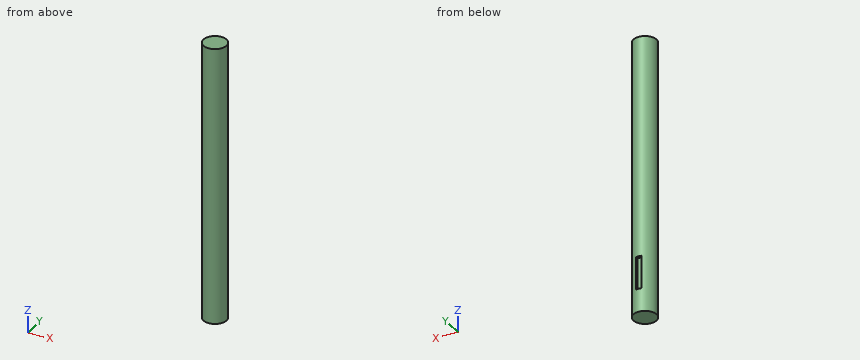
from build123d import *

# Parameters (mm, degrees)
SKETCH1_R           = 6.35
BOSS_EXTRUDE1_DEPTH = 152.4
CUT_EXTRUDE1_DEPTH  = 18.034


with BuildPart() as part:
    # Sketch1 → Boss-Extrude1 (new body)
    with BuildSketch(Plane.XY):
        with Locations(Location((0, 0, 0), (0, 0, 180))):
            Circle(SKETCH1_R)
    extrude(amount=BOSS_EXTRUDE1_DEPTH)

    # Sketch2 → Cut-Extrude1 (cut)
    with BuildSketch(Plane(origin=(0, 0, 12.7), x_dir=(-1, 0, 0), z_dir=(0, 0, -1))):
        Polygon((1.571433325, 4.7625), (-0.016066675, 4.7625), (-1.603566675, 4.7625), (-1.603566675, 7.9375), (1.571433325, 7.9375), align=None)
    extrude(amount=-CUT_EXTRUDE1_DEPTH, mode=Mode.SUBTRACT)


solid = part.part
Part model, mm, in its own coordinate system. Give positions to 0.01 mm unless a question says otherwise; leave off trailing zeros. Write each loop counter-clockwise with the first axis right and the second up, starting at its lowest first coordinate (ties: lowest second). Pieces come first, ordered by that corner, then holes.
1) Cut at A-A on z = 129. Write the cut outline in (x, y).
Resolved:
outline: circle Ø12.7 at (0, 0)
2) Probe L1, parallel to Y at x = 0.5, z = 121.5; L2, parallel to X at y = -4.5, z = 93.5; L3, parallel to Y at x = 2.5, z = 79. List the from-to ranges inside material, lowest first.
Resolved:
L1: y = -6.33 to 6.33
L2: x = -4.48 to 4.48
L3: y = -5.84 to 5.84
3) Cut at C-C on y = -3.25. Write the cut outline in (x, z), then the cut area to 3 significant figures.
Resolved:
outline: (-5.46, 0) - (5.46, 0) - (5.46, 152.4) - (-5.46, 152.4) - close
area: 1,660 mm2
4) Cut at B-B on x = -0.25. Write the cut outline in (y, z).
Resolved:
outline: (-6.35, 0) - (6.35, 0) - (6.35, 12.7) - (4.76, 12.7) - (4.76, 30.73) - (6.35, 30.73) - (6.35, 152.4) - (-6.35, 152.4) - close
5) Pin check, flat tips, straight feed: pin 1 (2 mm diameter, centred on x = 4, z = 43.5, fed in from -Y); pin 2 (5 mm diameter, centred on y = 3.5, z = 33.5, fed in from +X); pin 3 (0.5 mm diameter, centred on x = -0.5, y = 6, fed in from -Z); pin 4 (5 mm diameter, centred on x = 5, z = 135, fed in from +Y). Stop position of each tip, or through.
Resolved:
pin 1: stops at y = -5.6
pin 2: stops at x = 6.27
pin 3: stops at z = 0
pin 4: stops at y = 5.84
